Part print with two shaded views. Sizes in mm from the minimum x, y, z corner. A direction names the side the tool comes from. Coordinates: 2 decimals unless noted, no trailing zeros. Order: outer loops, then holes, each group sorted by start corner. A loop starts at its lowest first (then second) coordinate and runs counter-clockwise, first axis right, second up. Notation, with made-up numbers: (-7, -7.5) - (45, -7.5) arc R17 ccw to (45, 5.5) - close; hole circle Ø1 at (33, 81). An arc over 180 degrees is marked (long way). One line per item, written item: value.
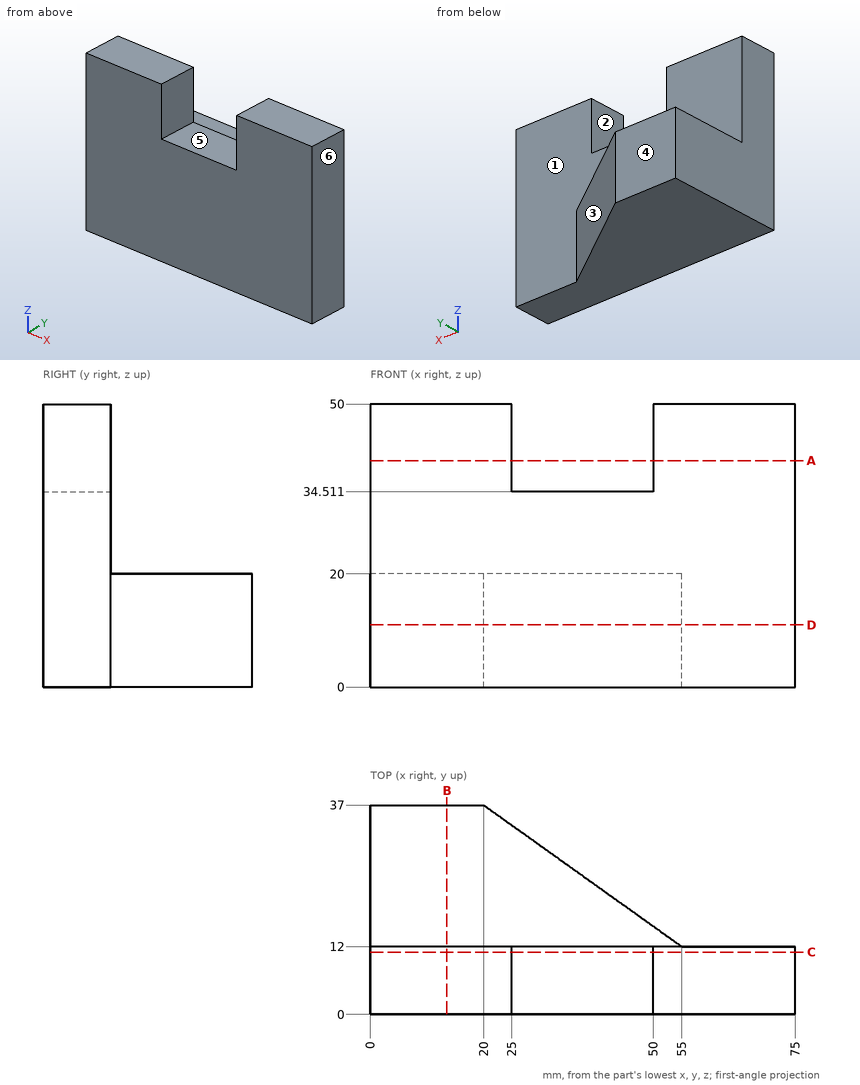
1. Band-saw the part on B-B, the plane x = 13.5. Give the cut face in (y, z), and give its area (3 significant figures).
Values found:
outline: (0, 0) - (37, 0) - (37, 20) - (12, 20) - (12, 50) - (0, 50) - close
area: 1,100 mm2
2. Band-saw the part on C-C, the plane y = 11. Give the cut face in (x, z), and give its area (3 significant figures).
Values found:
outline: (0, 0) - (75, 0) - (75, 50) - (50, 50) - (50, 34.51) - (25, 34.51) - (25, 50) - (0, 50) - close
area: 3,360 mm2
3. 3-axis set-ups, long thin cutter, end or side, ignore diameter. For the marked faces 1, 2 and 3: which of +Z, -Z, +X, -X, +Y, -Y reach the whole face in a straight line?
Values found:
face 1: +Z, +X, +Y
face 2: +Z, +Y, -Y
face 3: +Z, -Z, +X, +Y
4. Two-plate mould, pull along X, no slides. Class the marked faces 4, 5 and 6: pulls with the +X half, pulls with the -X half, needs draft (parallel to the pull), parting line crosses it, or undercut.
Values found:
face 4: needs draft
face 5: undercut
face 6: pulls with the +X half
5. Band-saw the part on D-D, the plane z = 11. Give the cut face in (x, y), and give its area (3 significant figures).
Values found:
outline: (0, 0) - (75, 0) - (75, 12) - (55, 12) - (20, 37) - (0, 37) - close
area: 1,840 mm2
6. Probe line 1 along X through (y, z) = (11, 48.5); line 2 along Z through (x, y) = (36, 11.5); line 3 along Z through (x, y) = (14, 33). List the from-to ranges inside material, lowest first.
Values found:
line 1: x = 0 to 25, 50 to 75
line 2: z = 0 to 34.51
line 3: z = 0 to 20
7. Flat gauge pins, fed straight in: P1, Ø6, axis at x = 35, y = 8, coming from the +Z side; P2, Ø7.5, axis at x = 37.5, y = 22, coming from the +Z side; P3, Ø12, axis at x = 46.5, z = 44.5, coming from the +Y side. Where does each tip first touch, or does it go through?
Values found:
P1: stops at z = 34.51
P2: stops at z = 20
P3: stops at y = 12
8. Band-saw the part on A-A, the plane z = 40. Give the cut face in (x, y), and give its area (3 significant figures).
Values found:
outline: (0, 0) - (25, 0) - (25, 12) - (0, 12) - close; (50, 0) - (75, 0) - (75, 12) - (50, 12) - close
area: 600 mm2
